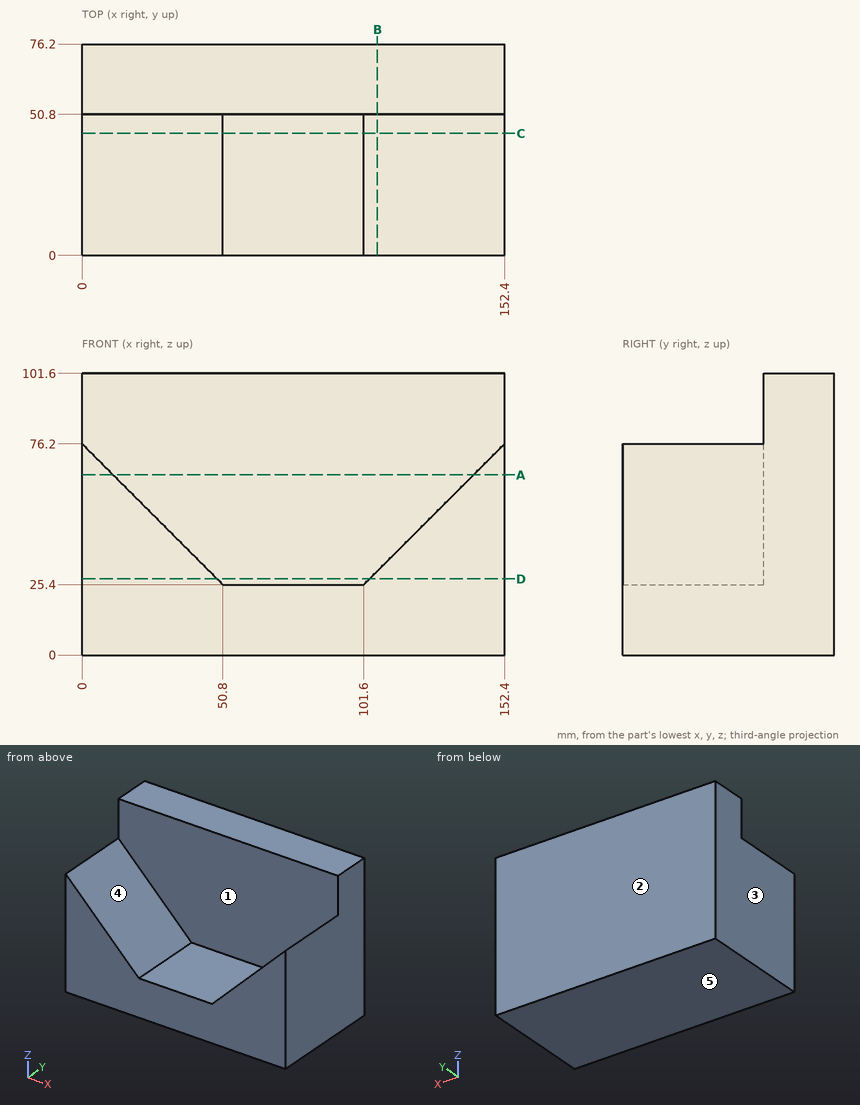
For this review, use the dimensioned drawing (mm, ordinates from the lowest corner) and the shaded views. A direction names the side the tool comes from. Coordinates: 2 decimals unless noted, no trailing zeros. Write each loop counter-clockwise with the first axis right and the second up, starting at its lowest first coordinate (ties: lowest second). Pieces come first, ordered by that corner, then holes. Notation, with made-up numbers: (43.25, 42.5) - (88.25, 42.5) arc R8 cw to (88.25, 49.5) - close; hole circle Ø10 at (48, 9). An arc over 180 degrees is marked (long way). Answer in a Markdown table with one row per item. Add a question column.
Q1. Draft analysis for pull direction X (two halves, no side actions). For the marked faces 3, 4 and 5, state which applies: +X half, -X half, draft (parallel to the pull), parting line (faces both ways), or undercut.
Q2. For the marked faces 1 and 2, list the 3-axis set-ups (+Z, -Z, +X, -X, +Y, -Y) from which the entire face can be reached by the end or side of a thin tool; tool diameter is ignored.
Q3. Consider section D-D on z = 27.5. Give the boundary of the cut face in (x, y), then the cut area to 3 significant figures.
Q4. Clearance check with a flat-ended pin moving along its axis: pin 1 (2 mm diameter, centred on x = 81.5, z = 46.5, fed in from -Y). State where the tip first meets the part, or that it passes through.
Q5. To check wall thickness, follow line 1 along Z through (x, y) = (67, 28.5); line 2 along Y through (x, z) = (24, 90); line 3 along X through (y, z) = (7, 71). State the ranges of each line that lie inside material, in increasing order. Write a range as from..to.
Q6. Consider section C-C on y = 44. Give the boundary of the cut face in (x, z).
Q7. Consider section B-B on x = 106.5. Give the boundary of the cut face in (y, z), then the cut area to 3 significant figures.
Q8. Consider section A-A on z = 65. Give the boundary of the cut face in (x, y), then the cut area to 3 significant figures.
Answers below:
| question | item | result |
|---|---|---|
| 1 | face 3 | -X half |
| 1 | face 4 | undercut |
| 1 | face 5 | draft |
| 2 | face 1 | +Z, -Y |
| 2 | face 2 | +Z, -Z, +X, -X, +Y |
| 3 | outline | (0, 0) - (48.7, 0) - (48.7, 50.8) - (103.7, 50.8) - (103.7, 0) - (152.4, 0) - (152.4, 76.2) - (0, 76.2) - close |
| 3 | area | 8,820 mm² |
| 4 | pin 1 | y = 50.8 |
| 5 | line 1 | 0..25.4 |
| 5 | line 2 | 50.8..76.2 |
| 5 | line 3 | 0..5.2, 147.2..152.4 |
| 6 | outline | (0, 0) - (152.4, 0) - (152.4, 76.2) - (101.6, 25.4) - (50.8, 25.4) - (0, 76.2) - close |
| 7 | outline | (0, 0) - (76.2, 0) - (76.2, 101.6) - (50.8, 101.6) - (50.8, 30.3) - (0, 30.3) - close |
| 7 | area | 4,120 mm² |
| 8 | outline | (0, 0) - (11.2, 0) - (11.2, 50.8) - (141.2, 50.8) - (141.2, 0) - (152.4, 0) - (152.4, 76.2) - (0, 76.2) - close |
| 8 | area | 5,010 mm² |
